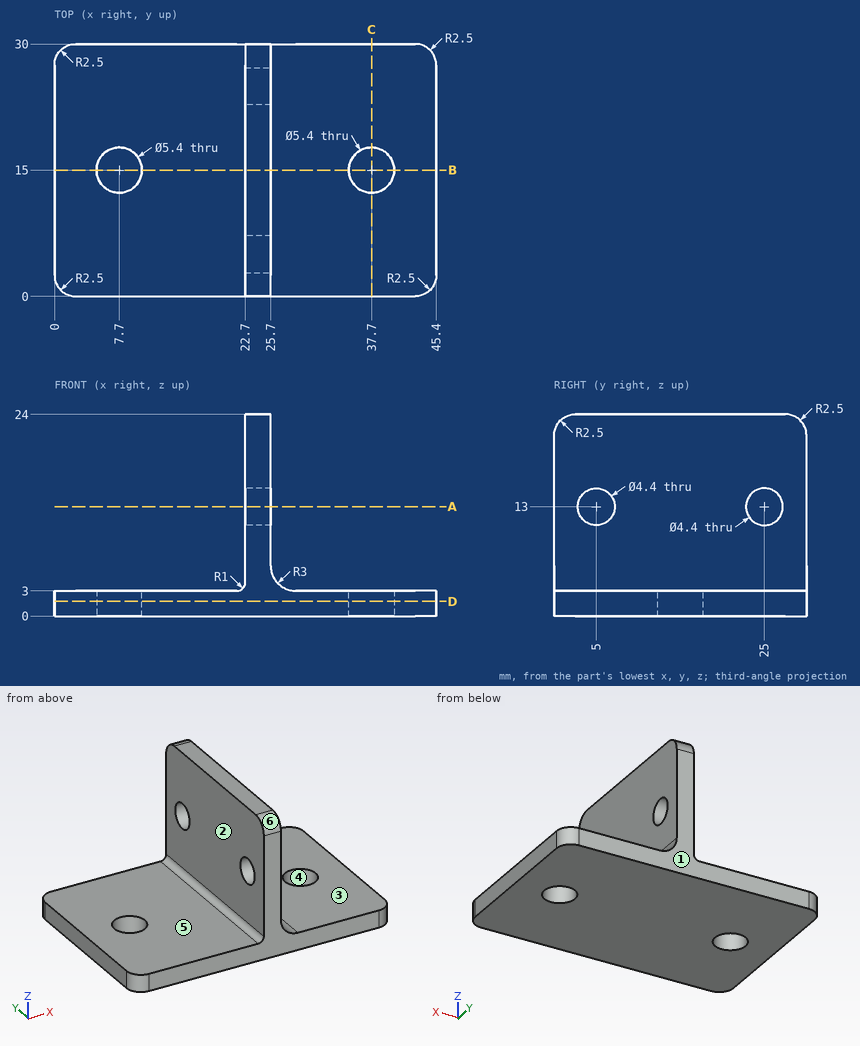
Can you work these out from the drawing? Everything is in mm from the part's minimum corner. A direction names the side the tool comes from. Give positions to 0.01 mm unless a question says otherwise; leave off trailing zeros. Order: outer loops, then holes, each group sorted by start corner. A loop starts at its lowest first (then second) coordinate and runs counter-clockwise, first axis right, second up. Notation, with made-up numbers: M 37,-35.75 L 48,-35.75 A25 ccw 48,-8.75 Z; hole C -13.5,3 d5. An arc over 180 degrees is marked long. Use a Markdown table: item, result. Add a question column.
1. Suppose I cut it at A-A (z = 13). List the corners of the cut face in (x, y) for me, and give its area (3 significant figures).
2. Suppose I cut it at C-C (x = 37.7). List the corners of the cut face in (y, z) for me.
3. For pin 1 Ø6 at (y, z) = (10, 13) entering from -X; pin 2 Ø6 at (y, z) = (23, 21.5) entering from +X; pin 3 Ø11 at (x, y) = (10.5, 16.5) entering from +Z, each with a flat end and sliding along its axis, tell me the tip position at first contact or that it passes through.
4. Suppose I cut it at B-B (y = 15). List the corners of the cut face in (x, z) for me, and give its area (3 significant figures).
5. If we mould it in two halves opening along Y, with no side actions, what happens to the marked faces 4, 5 and 6? For each: +Y half, -Y half, draft (parallel to the pull), parting line (faces both ways), or undercut.
6. Suppose I cut it at D-D (z = 1.75). List the corners of the cut face in (x, y) for me, and give its area (3 significant figures).
7. I need wall thicknesses on probe 1 along Y at (x, z) = (37.7, 1.5); probe 2 along Z at (x, y) = (24.65, 25); probe 3 along Z at (x, y) = (4, 18). Which ranges of each line are inside material? Lowest first, please. Write a range as from..to.
8. On a 3-axis mill with a long thin cutter (end or side, diameter ignored), from which of +Z, -Z, +X, -X, +Y, -Y can I reach the whole of each face in a straight line? I mean the marked faces 1, 2 and 3. Say none if no direction works.
Results list:
| question | item | result |
|---|---|---|
| 1 | outline | M 22.7,0 L 25.7,0 L 25.7,2.8 L 22.7,2.8 Z; M 22.7,7.2 L 25.7,7.2 L 25.7,22.8 L 22.7,22.8 Z; M 22.7,27.2 L 25.7,27.2 L 25.7,30 L 22.7,30 Z |
| 1 | area | 63.6 mm² |
| 2 | outline | M 0,0 L 12.3,0 L 12.3,3 L 0,3 Z; M 17.7,0 L 30,0 L 30,3 L 17.7,3 Z |
| 3 | pin 1 | stops at x = 22.7 |
| 3 | pin 2 | stops at x = 25.7 |
| 3 | pin 3 | stops at z = 3 |
| 4 | outline | M 0,0 L 5,0 L 5,3 L 0,3 Z; M 10.4,0 L 35,0 L 35,3 L 28.7,3 A3 cw 25.7,6 L 25.7,24 L 22.7,24 L 22.7,4 A1 cw 21.7,3 L 10.4,3 Z; M 40.4,0 L 45.4,0 L 45.4,3 L 40.4,3 Z |
| 4 | area | 169 mm² |
| 5 | face 4 | undercut |
| 5 | face 5 | draft |
| 5 | face 6 | -Y half |
| 6 | outline | M 0,2.5 A2.5 ccw 2.5,0 L 42.9,0 A2.5 ccw 45.4,2.5 L 45.4,27.5 A2.5 ccw 42.9,30 L 2.5,30 A2.5 ccw 0,27.5 Z; hole C 7.7,15 d5.4; hole C 37.7,15 d5.4 |
| 6 | area | 1,310 mm² |
| 7 | probe 1 | y = 0..12.3, 17.7..30 |
| 7 | probe 2 | z = 0..10.8, 15.2..24 |
| 7 | probe 3 | z = 0..3 |
| 8 | face 1 | +Z, -Z, +X, -X, +Y |
| 8 | face 2 | +Z, -X, +Y, -Y |
| 8 | face 3 | +Z, +X, +Y, -Y |
